from build123d import *

# Parameters (mm, degrees)
SKETCH_1_R      = 42
EXTRUDE_1_DEPTH = 30
EXTRUDE_2_DEPTH = 5


with BuildPart() as part:
    # Sketch 1 → Extrude 1 (new body)
    with BuildSketch(Plane.XY):
        Circle(SKETCH_1_R)
    extrude(amount=EXTRUDE_1_DEPTH)



with BuildPart() as body_2:
    # Sketch 2 → Revolve 1 (revolve)
    with BuildSketch(Plane.XY.offset(30), mode=Mode.PRIVATE) as revolve_1_sk:
        with BuildLine():
            Line((100, 20), (100, 15))
            ThreePointArc((100, 15), (86.583592135, 6.708203932), (88, -9))
            Line((88, -9), (80, -9))
            Line((80, -9), (80, 20))
            Line((80, 20), (100, 20))
        make_face()
    revolve(revolve_1_sk.sketch.rotate(Axis((100, 22.717290725, 30), (0, -1, 0)), 270), axis=Axis((100, 22.717290725, 30), (0, -1, 0)))


with BuildPart() as part_1:
    add(part.part)

    add(body_2.part)  # Extrude 2 merges body 2
    # Sketch 3 → Extrude 2 (add, symmetric)
    with BuildSketch(Plane.XY.offset(30)):
        with BuildLine():
            Line((14.069453744, 39.573355574), (86, 14))
            Line((86, 14), (86, -3))
            Line((86, -3), (19.208719722, -37.350034627))
            ThreePointArc((19.208719722, -37.350034627), (-41.906577017, -2.79978619), (14.069453744, 39.573355574))
        make_face()
    extrude(amount=EXTRUDE_2_DEPTH, both=True)


solid = part_1.part
Can you work these out from the model? Positions are in its coordinate system, mm. A direction names the side the tool comes from. Give positions to 0.01 mm unless a question says otherwise; leave off trailing zeros. Write each loop counter-clockwise with the first axis right and the second up, starting at its lowest first coordinate (ties: lowest second). Pieces come first, ordered by that corner, then holes. Notation, with made-up numbers: M -30.5,-22.75 L 1.5,-22.75 A18 ccw 1.5,-5.75 Z; hole C 2,72.25 d2. An arc over 180 degrees is marked long. Answer in a Markdown table with one row per item. Add a question column.
Item 1: Imagine slicing it at A-A, the plane y = 0. Write out the boundary of the cut face in (x, z), plus the area to 3 significant figures.
Item 2: We'd pull the mould along X, two halves only. Please class faces 1 (the cylindrical face through (119.524, 5.703, 25.664)), 2 (the flat face through (109, -9, 21)): released by +X, released by -X, zero draft, split by the parting line, or undercut.
Item 3: For pin 1 Ø2 at (x, z) = (-24, 8.5) entering from -Y; pin 2 Ø12 at (x, y) = (40.5, 26.5) entering from +Z; pin 3 Ø2 at (x, z) = (53, 34.5) entering from -Y; pin 4 Ø12 at (x, z) = (2, 14) entering from -Y, each with a flat end and sliding along its axis, tell me the tip position at first contact or that it passes through.
Item 4: Please list where these lines run through material, in increasing order: L1, parallel to X at y = 11.5, z = 14.5; L2, parallel to X at y = 12.5, z = 30; L3, parallel to Z at x = -15, y = -26.5.
Item 5: On a 3-axis mill with a long thin cutter (end or side, diameter ignored), from which of +Z, -Z, +X, -X, +Y, -Y can I reach the whole of each face in a straight line? I mean faces 3 (the flat face through (20, 1, 35)), 4 (the flat face through (86, 1, 30)), 5 (the flat face through (100, 20, 30)). Say none if no direction works.
Item 6: Imagine slicing it at B-B, the plane x = 100. Write out the boundary of the cut face in (y, z), plus the area to 3 significant figures.
Item 7: Imagine slicing it at C-C, the plane y = -33.5. Write out the boundary of the cut face in (x, z).
Item 8: Imagine slicing it at D-D, the plane x = 0. Write out the boundary of the cut face in (y, z).
Evaluation:
| question | item | result |
|---|---|---|
| 1 | outline | M -42,0 L 42,0 L 42,25 L 80.64,25 A20 ccw long 80.64,35 L -42,35 Z; hole M 85.86,25 A15 ccw long 85.86,35 L 86,35 L 86,25 Z |
| 1 | area | 3,880 mm² |
| 2 | face 1 | undercut |
| 2 | face 2 | zero draft |
| 3 | pin 1 | stops at y = -35.14 |
| 3 | pin 2 | stops at z = 35 |
| 3 | pin 3 | stops at y = -20.49 |
| 3 | pin 4 | stops at y = -42 |
| 4 | L1 | x = -40.39 to 40.39, 87.36 to 112.64 |
| 4 | L2 | x = -40.1 to 91.71, 108.29 to 120 |
| 4 | L3 | z = 0 to 35 |
| 5 | face 3 | +Z, -X, +Y, -Y |
| 5 | face 4 | none |
| 5 | face 5 | +Z, -Z, +X, +Y |
| 6 | outline | M -9,10 L 20,10 L 20,50 L -9,50 L -9,42 A15 cw long -9,18 Z |
| 6 | area | 554 mm² |
| 7 | outline | M -25.33,0 L 25.33,0 L 25.33,25 L 26.69,25 L 26.69,35 L -25.33,35 Z |
| 8 | outline | M -42,0 L 42,0 L 42,35 L -42,35 Z |
